Here's the drawing with two shaded views (mm, measured from the low corner). I have some questions. A direction names the side the tool comes from. Round coordinates to 2 decimals unless told otherwise and drop trailing zeros. Write each loop counter-clockwise with the first axis right and the second up, starting at its lowest first coordinate (ties: lowest second). Pieces come first, ordered by that corner, then holes. Notation, with made-up numbers: M -34,-31.5 L 11,-31.5 A10 ccw 11,-21.5 Z; hole C 50.25,-1.75 d1. An arc over 180 degrees is marked long. Use one line per item in the form item = value. Start each with the question number.
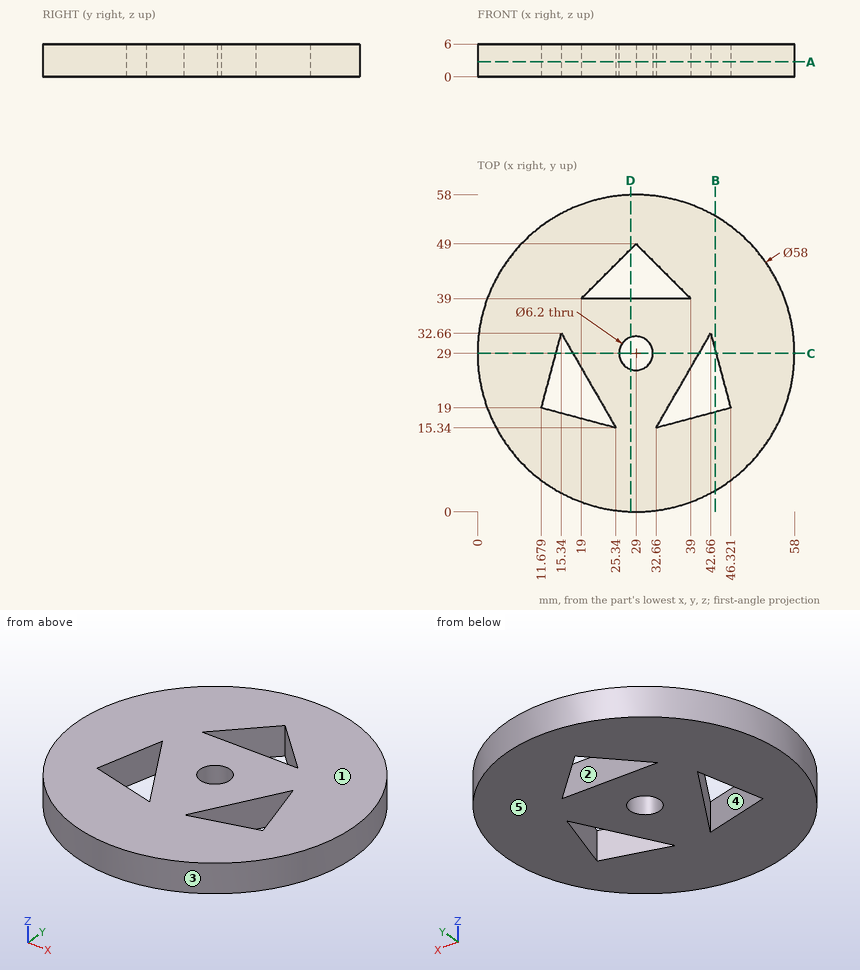
1. If we section it at D-D (x = 28): List the corners of the cut face in (y, z) for me (1 decimal).
2. If we section it at C-C (y = 29): List the corners of the cut face in (x, z) for me.
3. If we section it at A-A (z = 2.75): List the corners of the cut face in (x, y) for me, and give its area (3 significant figures).
4. Please list where these lines run through material, in increasing order: line 1 along Y through (x, z) = (37, 4.5) (1 decimal); line 2 along X through (y, z) = (31.5, 5.5) (1 decimal); line 3 along X through (y, z) = (30.5, 5.25) (1 decimal).
5. Will these pins go through, and if not, where does the flat tip stop? pin 1 (1.8 mm diameter, centred on x = 30, z = 2, fed in from +Y); pin 2 (1.5 mm diameter, centred on y = 22, z = 2.5, fed in from -X); pin 3 (1 mm diameter, centred on y = 36.5, z = 1.5, fed in from +X).
6. If we section it at B-B (x = 43.5): List the corners of the cut face in (y, z) for me (1 decimal).
7. Which directions (+Z, -Z, +X, -X, +Y, -Y) give clear straight access to the entire face, cutting with the end or side of a thin tool? Please do the marked faces 4 and 5.
8. If we mould it in two halves opening along Y, with no side actions, what happens to the marked faces 1, 2 and 3? For each: pulls with the +Y half, pulls with the -Y half, needs draft (parallel to the pull), parting line crosses it, or undercut.
Model answer:
q1.outline = M 0,0 L 26.1,0 L 26.1,6 L 0,6 Z; M 31.9,0 L 39,0 L 39,6 L 31.9,6 Z; M 48,0 L 58,0 L 58,6 L 48,6 Z
q2.outline = M 0,0 L 14.36,0 L 14.36,6 L 0,6 Z; M 17.45,0 L 25.9,0 L 25.9,6 L 17.45,6 Z; M 32.1,0 L 40.55,0 L 40.55,6 L 32.1,6 Z; M 43.64,0 L 58,0 L 58,6 L 43.64,6 Z
q3.outline = C 29,29 d58; hole M 11.68,19 L 25.34,15.34 L 15.34,32.66 Z; hole M 19,39 L 39,39 L 29,49 Z; hole C 29,29 d6.2; hole M 32.66,15.34 L 46.32,19 L 42.66,32.66 Z
q3.area = 2,310 mm2
q4.line_1 = 1.1 to 16.5, 22.9 to 39, 41 to 56.9
q4.line_2 = 0.1 to 15, 16 to 27.2, 30.8 to 42, 43 to 57.9
q4.line_3 = 0 to 14.8, 16.6 to 26.3, 31.7 to 41.4, 43.2 to 58
q5.pin_1 = 58
q5.pin_2 = 0.68
q5.pin_3 = 57.14
q6.outline = M 3.9,0 L 18.2,0 L 18.2,6 L 3.9,6 Z; M 29.5,0 L 54.1,0 L 54.1,6 L 29.5,6 Z
q7.face_4 = +Z, -Z
q7.face_5 = -Z, +X, -X, +Y, -Y
q8.face_1 = needs draft
q8.face_2 = undercut
q8.face_3 = parting line crosses it
